Geometry: see drawing. Coordinates: mm, zero at the bounding-box minimum. A direction names the side the tool comes from. Coordinates: 2 decimals unless noted, no trailing zeros. Write each loop counter-clockwise with the first axis right and the second up, starting at its lowest first coordinate (ties: lowest second). Pieces come first, ordered by that corner, then holes. Notation, with made-up numbers: (0, -21.5) -> (59, -21.5) arc R22 ccw to (59, 4.5) -> close; hole circle Ø7 at (64.25, -37). An arc over 180 degrees is marked (long way). Answer as a JSON object with one key per item and string values. Group by question number.
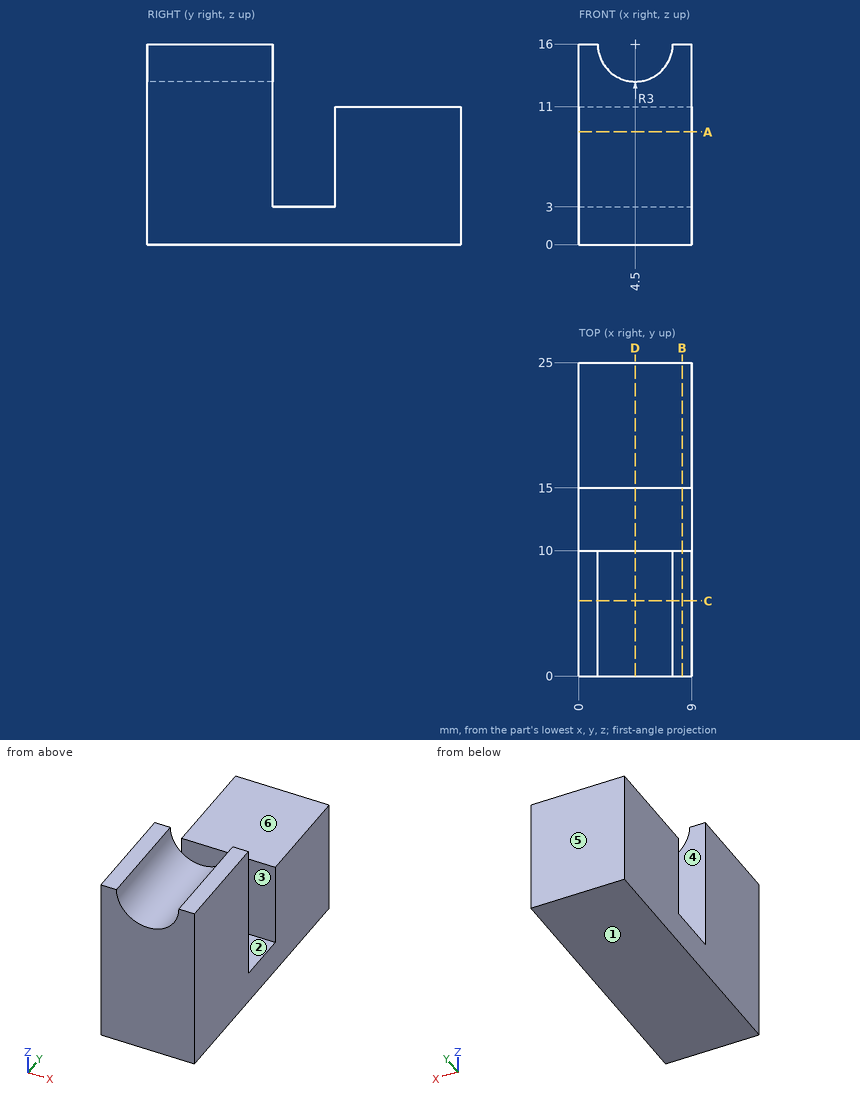
Item 1: Mould query, pull axis Y, two halves, no side actions, for the marked faces 3, 4, 5 and 6. Classes: +Y half, -Y half, draft (parallel to the pull), parting line (faces both ways), or undercut.
Item 2: Ray query, L1, parallel to Y at x = 2.25, z = 5; L2, parallel to Z at x = 0.75, y = 17; L3, parallel to Z at x = 8.5, y = 10.25. Return the intervals inside material, ascending. Write a range as [from, to].
Item 3: Set-up query: the marked faces 1 and 2. Return all of +Z, -Z, +X, -X, +Y, -Y with unobstructed straight access to the full face (end or side cutting, diameter ignored); none if empty.
Item 4: Section D-D on x = 4.5. Output: boundary loops of the cut face in (y, z), then the cut area to 3 significant figures.
Item 5: Section B-B on x = 8.25. Output: boundary loops of the cut face in (y, z), then the cut area to 3 significant figures.
Item 6: Contact query for a flat-ended pin moving along its axis: pin 1 (2 mm diameter, centred on x = 3.5, y = 19.5, fed in from +Z). Output: stop coordinate, or through.
Item 7: Section A-A on z = 9. Output: boundary loops of the cut face in (x, y).
Item 8: Section C-C on y = 6. Output: boundary loops of the cut face in (x, z), then the cut area to 3 significant figures.
Answer sheet:
{
 "1": {"face 3": "undercut", "face 4": "undercut", "face 5": "+Y half", "face 6": "draft"},
 "2": {"L1": "y = [0, 10], [15, 25]", "L2": "z = [0, 11]", "L3": "z = [0, 3]"},
 "3": {"face 1": "-Z, +X, -X, +Y, -Y", "face 2": "+Z, +X, -X"},
 "4": {"outline": "(0, 0) -> (25, 0) -> (25, 11) -> (15, 11) -> (15, 3) -> (10, 3) -> (10, 13) -> (0, 13) -> close", "area": "255 mm^2"},
 "5": {"outline": "(0, 0) -> (25, 0) -> (25, 11) -> (15, 11) -> (15, 3) -> (10, 3) -> (10, 16) -> (0, 16) -> close", "area": "285 mm^2"},
 "6": {"pin 1": "stops at z = 11"},
 "7": {"outline": "(0, 0) -> (9, 0) -> (9, 10) -> (0, 10) -> close; (0, 15) -> (9, 15) -> (9, 25) -> (0, 25) -> close"},
 "8": {"outline": "(0, 0) -> (9, 0) -> (9, 16) -> (7.5, 16) arc R3 cw to (1.5, 16) -> (0, 16) -> close", "area": "130 mm^2"}
}
